The figure shows three views and two pictorial views of one solid part (mm, origin at its lowest corner). Answer the questions. Coordinates: 2 decimals unless noted, no trailing zeros. Loops run counter-clockwise (first coordinate to the right, second up) from the corner with the lowest first, then second, coordinate; pieces in that order, holes last. Notation, with made-up numbers: M -19,-37.75 L 27,-37.75 A31 ccw 27,-12.75 Z; hole C -6,23 d5. An arc over 180 degrees is marked long. Write each question's results on one line, items separated by ' | '.
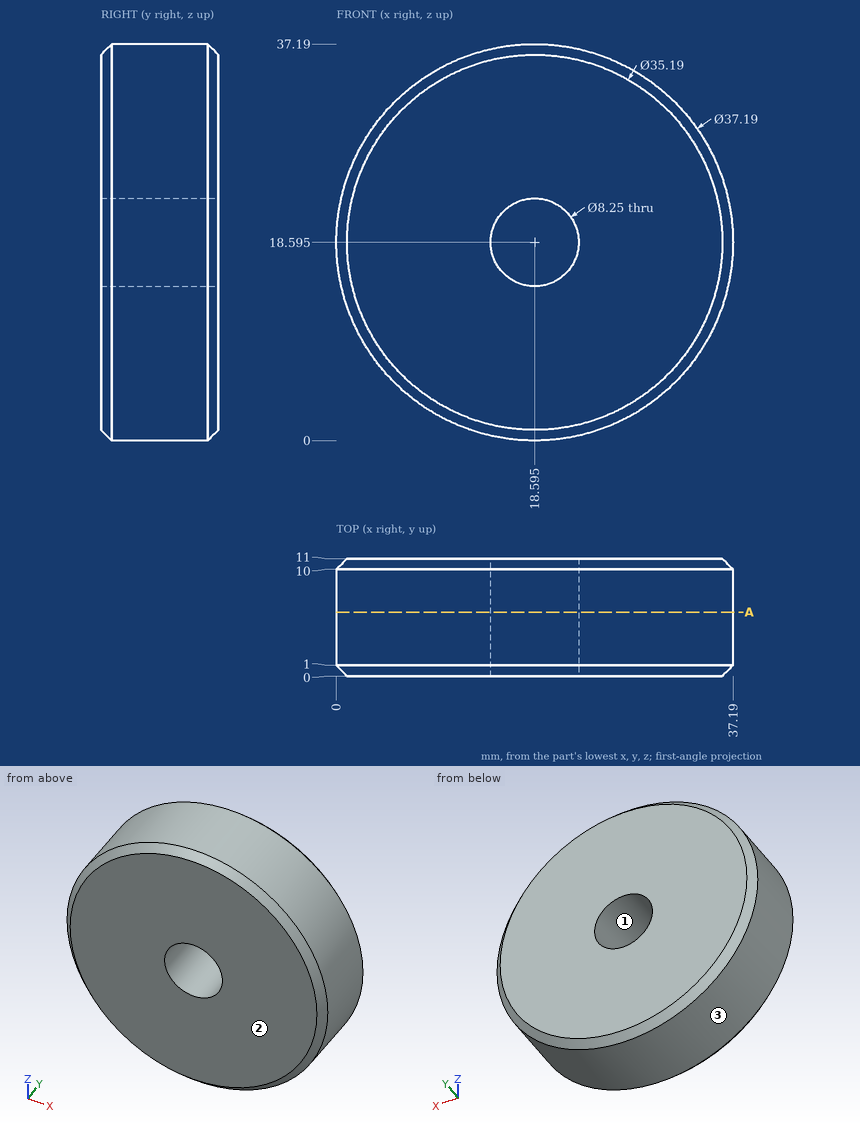
1) For a pull along X with two mould halves and no side action, classify the marked faces 1, 2 and 3 as released by +X, released by -X, zero draft, split by the parting line, or undercut.
Check result:
face 1: undercut | face 2: zero draft | face 3: split by the parting line
2) Find section A-A, the plane y = 6. Give the vertices of the cut face in (x, z) (3 decimals).
Check result:
outline: C 18.595,18.595 d37.19; hole C 18.595,18.595 d8.25
3) Straight lines are drawn through the part: probe 1 along Z at (x, y) = (15, 0.75); probe 2 along Z at (x, y) = (15.5, 10); probe 3 along X at (y, z) = (9.5, 10.5). For each, find the intervals that lie inside material, in ascending order. Write a range as [from, to].
Check result:
probe 1: [0.61, 16.57], [20.62, 36.58] | probe 2: [0.26, 15.87], [21.32, 36.93] | probe 3: [1.85, 35.34]
4) Given pin 1 Ø3 at (x, y) = (28.5, 4.5) entering from +Z; pin 2 Ø5 at (x, y) = (13.5, 7) entering from -Z; pin 3 Ø4 at (x, y) = (17, 5.5) entering from -Z, each flat-ended and moving along its own axis, determine where each tip first touches the part or whether it passes through.
Check result:
pin 1: z = 35.18 | pin 2: z = 0.18 | pin 3: z = 0
